```python
from build123d import *

# Parameters (mm, degrees)
F0_W     = 120
F0_H     = 120
F1_DEPTH = 19.5
F2_R     = 40
F3_DEPTH = 10
F4_W     = 20
F4_H     = 20
F6_DEPTH = 9


with BuildPart() as f1:
    # F0 (on Top) → F1 (new body)
    with BuildSketch(Plane.XY):
        with Locations((60, 60)):
            Rectangle(F0_W, F0_H)
    extrude(amount=F1_DEPTH)

    # F2 (on face) → F3 (cut)
    with BuildSketch(Plane.XY.offset(19.5)):
        with Locations((60, 60)):
            Circle(F2_R)
    extrude(amount=-F3_DEPTH, mode=Mode.SUBTRACT)

    # F4 (on face) → F6 (join)
    with BuildSketch(Plane.XY.offset(9.5)):
        with Locations((60, 60)):
            Rectangle(F4_W, F4_H)
    extrude(amount=F6_DEPTH)


solid = f1.part
```
Geometry: final body of the model. Coordinates: model frame, mm. A direction names the side the tool comes from. Give positions to 0.01 mm unless a question says otherwise; leave off trailing zeros. Write each loop counter-clockwise with the first axis right and the second up, starting at its lowest first coordinate (ties: lowest second). Pieces come first, ordered by that corner, then holes.
1. Section query B-B, the plane y = 60. Return loops of the section in (x, z), then the cut area to 3 significant figures.
2. Draft query along X for faces 3 (the flat face through (59, 101, 19.5)), 4 (the flat face through (60, 70, 14)), 5 (the flat face through (70, 60, 14)), 6 (the flat face through (120, 59, 10)). Return one class per face: released by +X, released by -X, zero draft, split by the parting line, or undercut.
3. Reachability of faces 1 (the flat face through (0, 59, 10)), 2 (the cylindrical face through (98.153, 72.015, 14.57)) from +Z, -Z, +X, -X, +Y, -Y: full face, straight path, thin tool, end or side. Return the list, or none.
4. Section query D-D, the plane y = 22. Return loops of the section in (x, z), then the cut area to 3 significant figures.
5. Section query A-A, the plane z = 15.5. Return loops of the section in (x, y).
6. Line query: probe 1 along Y at (x, z) = (60, 16); probe 2 along X at (y, z) = (51.5, 13.25); probe 3 along Y at (x, z) = (67, 16.75). Output: solid intervals per line, ascending.
7. Pin query (flat end, axial travel): P1, Ø2, axis at x = 84.5, y = 108, coming from the -Z side; P2, Ø24, axis at x = 64, y = 56, coming from the +Z side. Return the tip coordinate at first contact, or that it passes through.
Computed:
1. outline: (0, 0) - (120, 0) - (120, 19.5) - (100, 19.5) - (100, 9.5) - (70, 9.5) - (70, 18.5) - (50, 18.5) - (50, 9.5) - (20, 9.5) - (20, 19.5) - (0, 19.5) - close
1. area: 1,720 mm2
2. face 3: zero draft
2. face 4: undercut
2. face 5: undercut
2. face 6: released by +X
3. face 1: +Z, -Z, -X, +Y, -Y
3. face 2: +Z
4. outline: (0, 0) - (120, 0) - (120, 19.5) - (72.49, 19.5) - (72.49, 9.5) - (47.51, 9.5) - (47.51, 19.5) - (0, 19.5) - close
4. area: 2,090 mm2
5. outline: (0, 0) - (120, 0) - (120, 120) - (0, 120) - close; (50, 50) - (70, 50) - (70, 70) - (50, 70) - close; hole circle Ø80 at (60, 60)
6. probe 1: y = 0 to 20, 50 to 70, 100 to 120
6. probe 2: x = 0 to 20.91, 50 to 70, 99.09 to 120
6. probe 3: y = 0 to 20.62, 50 to 70, 99.38 to 120
7. P1: stops at z = 0
7. P2: stops at z = 18.5
